CAD build for the part. Positions are in the model's coordinates, mm. A direction names the side the tool comes from. Round coordinates to 2 decimals unless told otherwise and drop trailing zeros. Order: outer loops, then holes, each group sorted by start corner. A loop starts at its lowest first (then second) coordinate and runs counter-clockwise, first axis right, second up. Notation, with made-up numbers: (15.25, -7) -> (19.25, -7) arc R24 cw to (19.25, 20) -> close; hole circle Ø9 at (-18, 17.5). An arc over 180 degrees is marked (long way). Return JSON: item names as keys, results as strings. Group by question number.
Q1. Mould opens along X. For faces 4 (the flat face through (1, 2, 88.148)), 5 (the cylindrical face through (19.74, 1.01, 68.87)), 6 (the flat face through (-45, 2, 1)) say: +X half, -X half, draft (parallel to the pull), parting line (faces both ways), or undercut.
Q2. Which spindle directions (+Z, -Z, +X, -X, +Y, -Y) get a long thin tool onto all of the face, cutting with end or side? Do faces 1 (the flat face through (-38, 2, -88.148)), 2 (the cylindrical face through (-20.26, 1.01, 68.87)), 3 (the flat face through (37, 2, -88.148)). Say none if no direction does.
Q3. Cut at A-A (x = 20). Write the cut outline in (y, z), then the cut area to 3 significant figures.
Q4. Flat gauge pin, fed straight in: pin 1 (2 mm diameter, centred on x = 37.5, y = 3, fed in from -Z). Where does the tip first touch, or does it go through?
Q5. Probe line 1 along Z through (x, y) = (-20, 0.4); line 2 along Z through (x, y) = (-37, 1.85). List the from-to ranges inside material, lowest first.
Autodesk Inventor part; units mm, degrees
ref_plane "YZ Plane" through (0, 0, 0) normal (1, 0, 0) x (0, 1, 0)
ref_plane "XZ Plane" through (0, 0, 0) normal (0, 1, 0) x (-1, 0, 0)
ref_plane "XY Plane" through (0, 0, 0) normal (0, 0, 1) x (1, 0, 0)
sketch "Эскиз1" plane through (0, 0, 0) normal (0, 1, 0) x (-1, 0, 0)
  line L0 (-45, 88.1475) -> (45, 88.1475)
  line L1 (45, 88.1475) -> (45, -88.1475)
  line L2 (45, -88.1475) -> (-45, -88.1475)
  line L3 (-45, -88.1475) -> (-45, 88.1475)
  line L4 (-45, 88.1475) -> (45, -88.1475) construction
  line L5 (45, 88.1475) -> (-45, -88.1475) construction
  point P0 (0, 0)
  dimension "d0" = 90
  dimension "d1" = 176.295
extrude "Выдавливание1" add sketch "Эскиз1" along normal blind 4
sketch "Эскиз2" plane through (0, 4, 0) normal (0, 1, 0) x (1, 0, 0)
  circle A0 centre (-20, -70.8525) radius 2
  circle A1 centre (20, -70.8525) radius 2
  point P0 (0, 0)
extrude "Выдавливание2" cut sketch "Эскиз2" against normal through all
chamfer "Фаска1" distance 2 angle 45 2 edges at (-22, 4, 70.8525) (18, 4, 70.8525)
sketch "Эскиз3" plane through (45, 0, -88.1475) normal (0, 0, -1) x (-1, 0, 0)
  line L0 (90, 4) -> (0, 4)
  line L1 (90, 0) -> (0, 0)
  line L2 (15, 4) -> (75, 4)
  line L3 (75, 4) -> (75, 0)
  line L4 (75, 0) -> (15, 0)
  line L5 (15, 0) -> (15, 4)
  point P0 (45, 0)
  point P1 (45, 0)
  dimension "d9" = 60
  dimension "d10" = 30
extrude "Выдавливание3" add sketch "Эскиз3" along normal blind 5
properties part number "000.005.003 - Крышка"
Solution:
{
 "1": {"face 4": "draft", "face 5": "undercut", "face 6": "-X half"},
 "2": {"face 1": "-Z, -X, +Y, -Y", "face 2": "+Y, -Y", "face 3": "-Z, +X, +Y, -Y"},
 "3": {"outline": "(0, -93.15) -> (4, -93.15) -> (4, 66.85) -> (2, 68.85) -> (0, 68.85) -> close; (0, 72.85) -> (2, 72.85) -> (4, 74.85) -> (4, 88.15) -> (0, 88.15) -> close", "area": "705 mm²"},
 "4": {"pin 1": "stops at z = -88.15"},
 "5": {"line 1": "z = -93.15 to 68.85, 72.85 to 88.15", "line 2": "z = -88.15 to 88.15"}
}
